For this review, use the dimensioned drawing (mm, ordinates from the lowest corner) and the shaded views. A direction names the side the tool comes from. Coordinates: 2 decimals unless noted, no trailing zeros. Write each loop counter-clockwise with the first axis right and the second up, starting at its lowest first coordinate (ties: lowest second). Pieces come first, ordered by that corner, then holes. Notation, with made-up numbers: (83, 75) - (138, 75) arc R26 cw to (138, 113) - close; hole circle Ø7 at (87.25, 49). An arc over 180 degrees is marked (long way). Put each result on its own line as item: value.
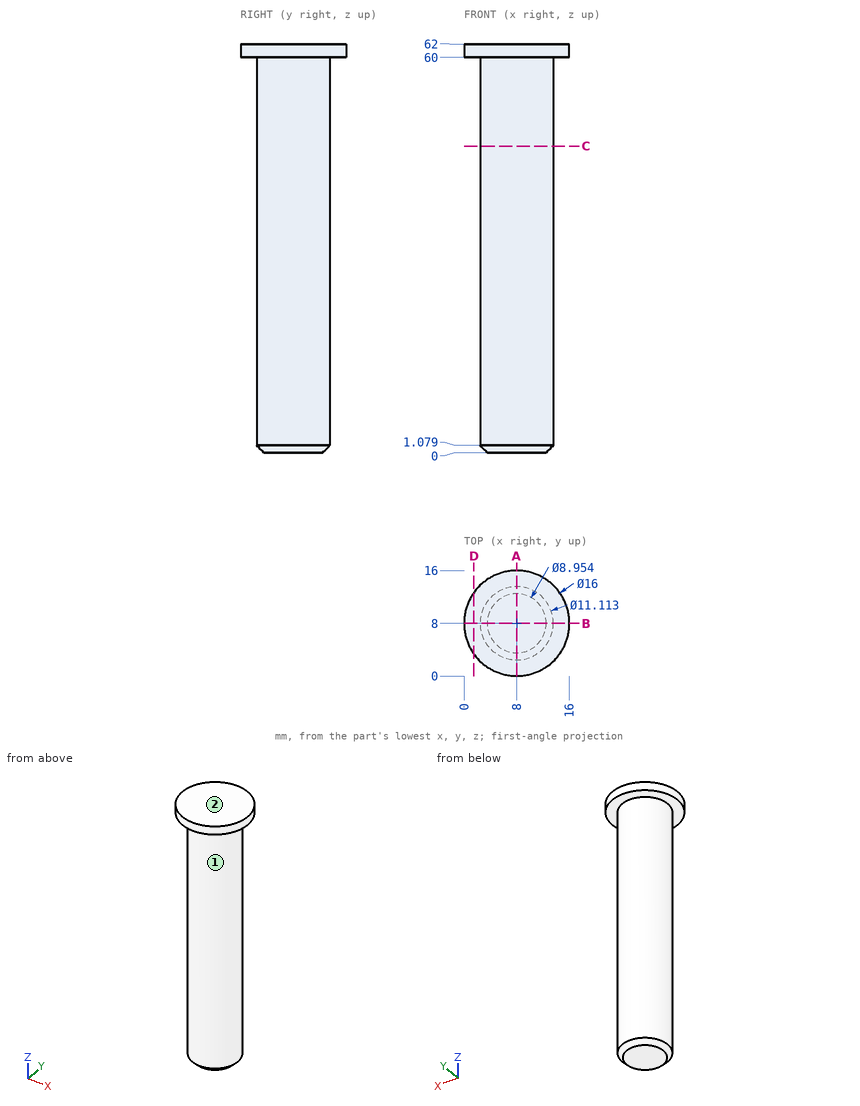
1. Consider section D-D on x = 1.5. State the section outline as (y, z) points.
Determined:
outline: (3.34, 60) - (12.66, 60) - (12.66, 62) - (3.34, 62) - close
2. Consider section A-A on x = 8. State the section outline as (y, z) points.
Determined:
outline: (0, 60) - (2.44, 60) - (2.44, 1.08) - (3.52, 0) - (12.48, 0) - (13.56, 1.08) - (13.56, 60) - (16, 60) - (16, 62) - (0, 62) - close
3. To check wall thickness, follow probe 1 along Z at (x, y) = (6.75, 14.5); probe 2 along Y at (x, z) = (8.25, 38.5). State the ranges of each line that lie inside material, in increasing order.
Determined:
probe 1: z = 60 to 62
probe 2: y = 2.45 to 13.55
4. Consider section C-C on z = 46.5. State the section outline as (x, y) points.
Determined:
outline: circle Ø11.11 at (8, 8)
5. For pin 1 Ø2 at (y, z) = (9, 13.5) entering from +X; pin 2 Ø8 at (x, y) = (9, 10) entering from -Z; pin 3 Ø2 at (y, z) = (5, 13.5) entering from -X, all flat-tipped, find the tip position at first contact; note any pin that passes through.
Determined:
pin 1: stops at x = 13.56
pin 2: stops at z = 0
pin 3: stops at x = 2.82
6. Machinability: for the marked faces 1 and 2, which of the approach directions +Z, -Z, +X, -X, +Y, -Y give a long, thin tool a straight path to every point of the face, cutting with its end or side? Answer none if there is none.
Determined:
face 1: -Z
face 2: +Z, +X, -X, +Y, -Y
